Input: dimensioned drawing with shaded views. Units: mm. Origin: part minimum x, y, z. A direction names the side the tool comes from. Coordinates: 2 decimals unless noted, no trailing zeros. Loops run counter-clockwise (first coordinate to the right, second up) from the corner with the lowest first, then second, coordinate; pieces in that order, holes last.
Item 1: Section query A-A, the plane z = 181. Return the cut outline in (x, y) (1 decimal).
Item 2: Pull-direction query (X, two-part tool) for the marked faces 1 and 2; classes: +X half, -X half, draft (parallel to the pull), parting line (faces both ways), or undercut.
Item 3: Pin query (flat end, axial travel): pin 1 Ø2 at (x, z) = (584, 345) entering from +Y; pin 2 Ø4 at (y, z) = (668, 125.5) entering from -X; pin 3 Ø12 at (y, z) = (184, 394) entering from +X. Return the tip coordinate at first contact, or that it passes through.
Item 4: Reachability of the marked faces 3 and 4 from +Z, -Z, +X, -X, +Y, -Y: full face, straight path, thin tool, end or side. Return the list, or none.
Item 5: Line query: probe 1 along Z at (x, y) = (532, 407); probe 2 along Y at (x, z) = (684, 118.5) (1 decimal); probe 3 along X at (y, z) = (324, 55.5) (1 decimal). Output: solid intervals per line, ascending.
Item 6: Section query C-C, the plane z = 332.5. Return the cut outline in (x, y) (1 decimal), then the cut area to 3 significant figures.
Item 7: Section query B-B, the plane z = 256.5. Return the cut outline in (x, y).
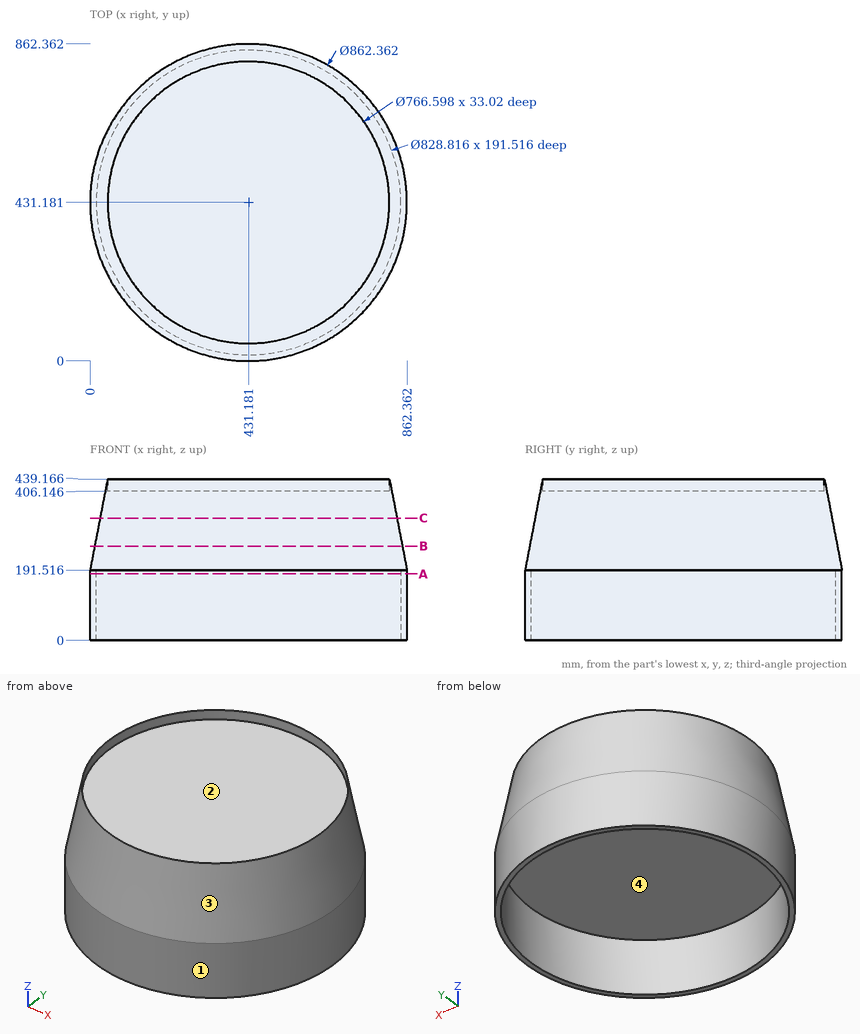
Verdict:
1. outline: circle Ø862.4 at (431.2, 431.2); hole circle Ø828.8 at (431.2, 431.2)
2. face 1: parting line
2. face 2: undercut
3. pin 1: stops at y = 802.93
3. pin 2: stops at x = 69.55
3. pin 3: stops at x = 740.47
4. face 3: +Z
4. face 4: -Z
5. probe 1: z = 191.52 to 406.15
5. probe 2: y = 81.9 to 102.8, 759.5 to 780.5
5. probe 3: x = 13.5 to 30.9, 831.5 to 848.8
6. outline: circle Ø807.8 at (431.2, 431.2)
6. area: 513,000 mm2
7. outline: circle Ø837.23 at (431.18, 431.18)
